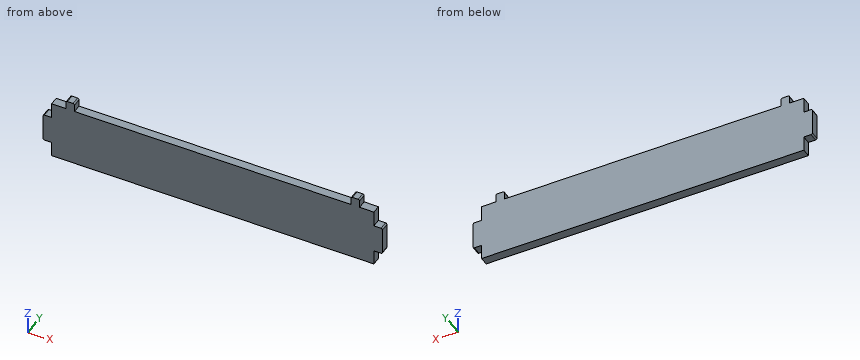
```python
from build123d import *

# Parameters (mm, degrees)
SKETCH_1_W      = 3
SKETCH_1_H      = 3
EXTRUDE_1_DEPTH = 3
FILLET_1_R      = 0.5


with BuildPart() as part:
    # Эскиз1 → Бобышка-Вытянуть1 (new body)
    with BuildSketch(Plane(origin=(0, 0, 0), x_dir=(1, 0, 0), z_dir=(0, 1, 0))):
        Polygon((-56.25, -20.75), (56.25, -20.75), (56.25, -15.25), (59.25, -15.25), (59.25, -5.25), (56.25, -5.25), (56.25, 0), (-56.25, 0), (-56.25, -5.25), (-59.25, -5.25), (-59.25, -15.25), (-56.25, -15.25), align=None)
        with Locations((49.75, -22.25)):
            Rectangle(SKETCH_1_W, SKETCH_1_H)
        with Locations((-49.75, -22.25)):
            Rectangle(SKETCH_1_W, SKETCH_1_H)
    extrude(amount=EXTRUDE_1_DEPTH)

    # Скругление1
    fillet_1_edges = [part.edges().sort_by_distance(p)[0] for p in [
        (-59.25, 1.5, 15.25),
        (-59.25, 1.5, 5.25),
        (59.25, 1.5, 5.25),
        (59.25, 1.5, 15.25),
        (51.25, 1.5, 23.75),
        (48.25, 1.5, 23.75),
        (-48.25, 1.5, 23.75),
        (-51.25, 1.5, 23.75),
    ]]
    fillet(fillet_1_edges, radius=FILLET_1_R)


solid = part.part
```
Work out the finished part from the listing and answer in its coordinate system (mm). Round coordinates to 2 decimals unless told otherwise and drop trailing zeros. Loops run counter-clockwise (first coordinate to the right, second up) from the corner with the lowest first, then second, coordinate; pieces in that order, holes last. Notation, with made-up numbers: M 11.5,-12.75 L 69.5,-12.75 A12 cw 69.5,-5.75 Z; hole C 27.25,83.5 d9. An arc over 180 degrees is marked long. Use CSV: the item, a comma, the result in double quotes.
Q1. Section C-C, the plane x = 21 is taken. Determine the outline of the cut face in (y, z), then the cut area to 4 significant figures.
Determined:
outline,"M 0,0 L 3,0 L 3,20.75 L 0,20.75 Z"
area,"62.25 mm2"
Q2. Section A-A, the plane y = 0.7 is taken. Determine the outline of the cut face in (x, z).
Determined:
outline,"M -59.25,5.75 A0.5 ccw -58.75,5.25 L -56.25,5.25 L -56.25,0 L 56.25,0 L 56.25,5.25 L 58.75,5.25 A0.5 ccw 59.25,5.75 L 59.25,14.75 A0.5 ccw 58.75,15.25 L 56.25,15.25 L 56.25,20.75 L 51.25,20.75 L 51.25,23.25 A0.5 ccw 50.75,23.75 L 48.75,23.75 A0.5 ccw 48.25,23.25 L 48.25,20.75 L -48.25,20.75 L -48.25,23.25 A0.5 ccw -48.75,23.75 L -50.75,23.75 A0.5 ccw -51.25,23.25 L -51.25,20.75 L -56.25,20.75 L -56.25,15.25 L -58.75,15.25 A0.5 ccw -59.25,14.75 Z"
Q3. Each of these flat-tipped pins is pushed along its axis until it touches: pin 1 (1.5 mm diameter, centred on y = 2, z = 2, fed in from +X); pin 2 (1.2 mm diameter, centred on x = -57, y = 1.5, fed in from +Z); pin 3 (1.5 mm diameter, centred on x = 45.5, y = 2, fed in from -Z); pin 4 (1.2 mm diameter, centred on y = 2, z = 22, fed in from -X). Where does it stop, or does it pass through?
Determined:
pin 1,"x = 56.25"
pin 2,"z = 15.25"
pin 3,"z = 0"
pin 4,"x = -51.25"
Q4. Consider L1, parallel to X at y = 0.45, z = 21.25; L2, parallel to X at y = 1.05, z = 2.25; L3, parallel to Z at x = 35, y = 2.85. Determine where each line is inside the solid, lowest interval first.
Determined:
L1,"-51.25 to -48.25, 48.25 to 51.25"
L2,"-56.25 to 56.25"
L3,"0 to 20.75"
Q5. Section B-B, the plane z = 17.75 is taken. Determine the outline of the cut face in (x, y).
Determined:
outline,"M -56.25,0 L 56.25,0 L 56.25,3 L -56.25,3 Z"
